Study the drawing (mm; zero at the part's minimum x, y, z) and answer. Give positions to 0.01 mm unless a question says otherwise; leave off trailing zeros. Loops run counter-clockwise (first coordinate to the right, second up) from the corner with the lowest first, then second, coordinate; pieces in that order, holes last. Notation, with made-up numbers: M -34.75,-19 L 7.25,-19 A17 cw 7.25,-11 Z; hole C -34,85 d10. An arc over 180 degrees is marked long. Return JSON: item names as keys, results as strings.
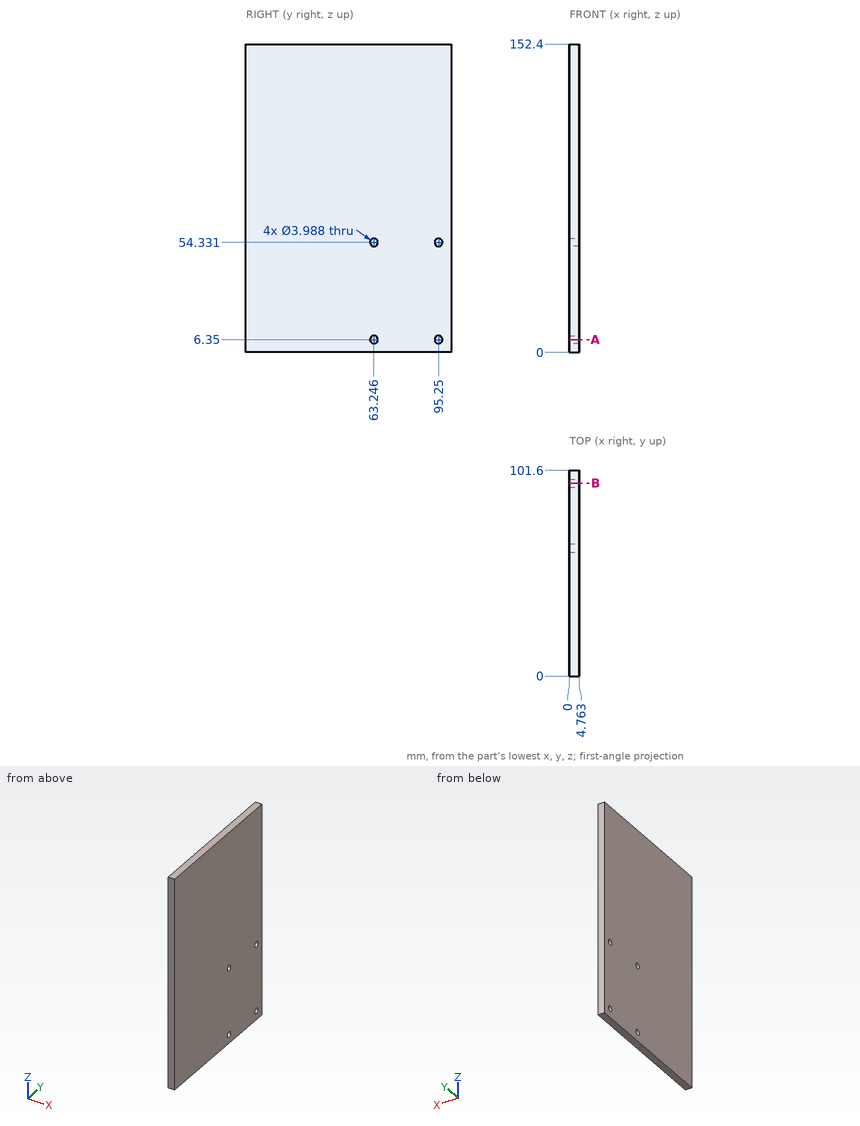
(1) The part is cut by section A-A (z = 6.35). Determine the outline of the cut face in (x, y), and give its area (3 significant figures).
Values follow:
{"outline": "M 0,0 L 4.76,0 L 4.76,61.25 L 0,61.25 Z; M 0,65.24 L 4.76,65.24 L 4.76,93.26 L 0,93.26 Z; M 0,97.24 L 4.76,97.24 L 4.76,101.6 L 0,101.6 Z", "area": "446 mm²"}
(2) Straight lines are drawn through the part: line 1 along Y through (x, z) = (2.55, 6.35); line 2 along Y through (x, z) = (1.65, 7.5) (1 decimal); line 3 along Z through (x, y) = (2.6, 97) (1 decimal). For each, find the intervals that lie inside material, in ascending order.
Values follow:
{"line 1": "0 to 61.25, 65.24 to 93.26, 97.24 to 101.6", "line 2": "0 to 61.6, 64.9 to 93.6, 96.9 to 101.6", "line 3": "0 to 5.4, 7.3 to 53.4, 55.3 to 152.4"}
(3) The part is cut by section B-B (y = 95.25). Determine the outline of the cut face in (x, z) (1 decimal).
Values follow:
{"outline": "M 0,0 L 4.8,0 L 4.8,4.4 L 0,4.4 Z; M 0,8.3 L 4.8,8.3 L 4.8,52.3 L 0,52.3 Z; M 0,56.3 L 4.8,56.3 L 4.8,152.4 L 0,152.4 Z"}
(4) Given pin 1 (4.5 mm diameter, centred on y = 95.25, z = 54.33, fed in from -X); pin 2 (3.5 mm diameter, centred on y = 63.25, z = 54.33, fed in from -X), each flat-ended and moving along its own axis, determine where each tip first touches the part or whether it passes through.
Values follow:
{"pin 1": "x = 0", "pin 2": "through"}
